```python
from build123d import *

# Parameters (mm, degrees)
BOSS_EXTRUDE1_DEPTH = 12.573


with BuildPart() as part:
    # Sketch1 → Boss-Extrude1 (new body)
    with BuildSketch(Plane(origin=(0, 0, 0), x_dir=(0, 0, -1), z_dir=(1, 0, 0))):
        with BuildLine():
            Line((0, 0), (0, 6.35))
            Line((0, 6.35), (3.175, 6.35))
            Line((3.175, 6.35), (3.175, 3.175))
            Line((3.175, 3.175), (30.1625, 3.175))
            Line((30.1625, 3.175), (30.1625, 0))
            Line((30.1625, 0), (26.9875, 0))
            Line((26.9875, 0), (26.9875, 0.889))
            ThreePointArc((26.9875, 0.889), (26.68992049, 1.60742049), (25.9715, 1.905))
            Line((25.9715, 1.905), (8.9535, 1.905))
            ThreePointArc((8.9535, 1.905), (8.23507951, 1.60742049), (7.9375, 0.889))
            Line((7.9375, 0.889), (7.9375, 0.635))
            ThreePointArc((7.9375, 0.635), (7.751512806, 0.185987194), (7.3025, 0))
            Line((7.3025, 0), (0, 0))
        make_face()
    extrude(amount=BOSS_EXTRUDE1_DEPTH)


solid = part.part
```
Work out the finished part from the listing and answer in its coordinate system (mm). A direction names the side the tool comes from. Round coordinates to 2 decimals unless told otherwise and drop trailing zeros. Loops run counter-clockwise (first coordinate to the right, second up) from the corner with the lowest first, then second, coordinate; pieces in that order, holes last. Notation, with made-up numbers: M -3.5,34.25 L 49.5,34.25 A12 ccw 49.5,43.25 Z; hole C 53.5,10 d1. An arc over 180 degrees is marked long. One line per question, with ' | ' between items.
Q1. Each of these flat-tipped pins is pushed along its axis until it touches: pin 1 Ø1.6 at (x, y) = (3.5, 5) entering from -Z (3 decimals); pin 2 Ø0.7 at (x, y) = (7.5, 0.5) entering from +Z; pin 3 Ø6.5 at (x, z) = (3.5, -19.5) entering from -Y (3 decimals); pin 4 Ø5 at (x, z) = (5.5, -12) entering from +Y (3 decimals). Where does it stop, or does it pass through?
Conclusion:
pin 1: stops at z = -3.175 | pin 2: stops at z = 0 | pin 3: stops at y = 1.905 | pin 4: stops at y = 3.175
Q2. Consider line 1 along Z through (x, y) = (7.5, 5.75) (3 decimals); line 2 along Y through (x, z) = (5.75, -14.5) (3 decimals); line 3 along Z through (x, y) = (5.75, 1.75). Determine where each line is inside the solid, lowest interval first. Write a range as from..to.
Conclusion:
line 1: z = -3.175..0 | line 2: y = 1.905..3.175 | line 3: z = -30.16..-26.51, -8.41..0
Q3. Find section C-C, the plane z = -9.5. Give the vertices of the cut face in (x, y) (3 decimals).
Conclusion:
outline: M 0,1.905 L 12.573,1.905 L 12.573,3.175 L 0,3.175 Z
Q4. The mould has two halves that part along Z. Classify faces 4 (the flat face through (6, 3.175, -16)), 5 (the flat face through (6.2, 0.4, -26.988)), 6 (the flat face through (6, 2, -30.162)): +Z half, -Z half, draft (parallel to the pull), parting line (faces both ways), or undercut.
Conclusion:
face 4: draft | face 5: undercut | face 6: -Z half
Q5. Find section D-D, the plane y = 5.25. Give the vertices of the cut face in (x, z) (3 decimals), then the cut area to 3 significant figures.
Conclusion:
outline: M 0,-3.175 L 12.573,-3.175 L 12.573,0 L 0,0 Z | area: 39.9 mm2
Q6. A tool of negligible diameter and unlimited length cuts with its end or side. For faces 1 (the flat face through (12.573, 2.5, -11.8)), 2 (the flat face through (6, 5, -3.175)), 3 (the cylindrical face through (6.198, 1.615, -8.243)), from which of +Z, -Z, +X, -X, +Y, -Y can it reach the whole face along a straight path? Write none if from no direction.
Conclusion:
face 1: +Z, -Z, +X, +Y, -Y | face 2: -Z, +X, -X, +Y | face 3: +X, -X, -Y
Q7. Find section A-A, the plane y = 1.25. Give the vertices of the cut face in (x, z), then the cut area to 3 significant figures.
Conclusion:
outline: M 0,-30.16 L 12.57,-30.16 L 12.57,-26.92 L 0,-26.92 Z; M 0,-8 L 12.57,-8 L 12.57,0 L 0,0 Z | area: 141 mm2
